Source: CAD feature listing. Evaluate the final solid. Frame: model axes, mm. Face numbers are marked on the shaded views. A direction names the side the tool comes from. Give positions to 0.01 mm unless a question says otherwise; leave off trailing zeros. Order: outer loops, then holes, each group sorted by start corner. A loop starts at its lowest first (then second) coordinate and runs counter-clockwise, first axis right, second up. Notation, with made-up numbers: (-10, 6.25) - (-6, 6.25) arc R3 ccw to (-6, 10.25) - close; hole circle Ø1 at (11, -19). An arc over 180 degrees is marked (long way). Use CSV: the item, a comma, the result in double quotes.
```python
from build123d import *

# Parameters (mm, degrees)
SKETCH_1_W               = 20
SKETCH_1_H               = 10
EXTRUDE_2_DEPTH          = 10
SKETCH_2_W               = 6
SKETCH_2_H               = 2
SKETCH_2_W_2             = 16
SKETCH_2_H_2             = 3
SKETCH_2_W_3             = 1.5
CUT_EXTRUDE_1_DEPTH      = 23.912878475
CUT_EXTRUDE_2_DEPTH      = 20
CUT_EXTRUDE_2_DEPTH_BACK = 20
SKETCH_7_W               = 17
SKETCH_7_H               = 5.873697418


with BuildPart() as part:
    # Эскиз1 → Бобышка-Вытянуть2 (new, symmetric)
    with BuildSketch(Plane.XY):
        Rectangle(SKETCH_1_W, SKETCH_1_H)
    extrude(amount=EXTRUDE_2_DEPTH, both=True)

    # Эскиз2 → Вырез-Вытянуть1 (cut, through all)
    with BuildSketch(Plane.XY.offset(10)):
        with Locations((-7, 4)):
            Rectangle(SKETCH_2_W, SKETCH_2_H)
        Polygon((10, 5), (3, 5), (10, -0.873697418), align=None)
        with Locations((-2, -3.5)):
            Rectangle(SKETCH_2_W_2, SKETCH_2_H_2)
        with Locations((9.25, -4)):
            Rectangle(SKETCH_2_W_3, SKETCH_2_H)
    extrude(amount=-CUT_EXTRUDE_1_DEPTH, mode=Mode.SUBTRACT)

    # Эскиз7 → Вырез-Вытянуть2 (cut, two sides: drawn at the far end of the back side and taken through both)
    with BuildSketch(Plane(origin=(0, 0, 0), x_dir=(0, 0, -1), z_dir=(1, 0, 0)).offset(-CUT_EXTRUDE_2_DEPTH_BACK)):
        with Locations((0, 2.063151291)):
            Rectangle(SKETCH_7_W, SKETCH_7_H)
    extrude(amount=CUT_EXTRUDE_2_DEPTH + CUT_EXTRUDE_2_DEPTH_BACK, mode=Mode.SUBTRACT)


solid = part.part
```
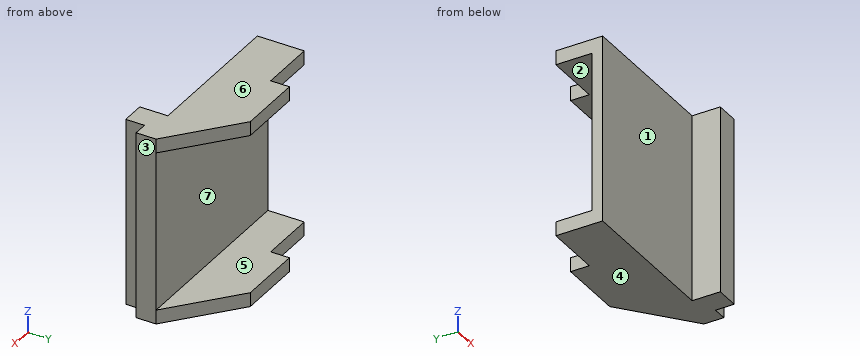
Item 1: Mould query, pull axis Z, two halves, no side actions, for the marked faces 4, 5, 6 and 7. Classes: released by +Z, released by -Z, zero draft, split by the parting line, or undercut.
Filled in:
face 4,"released by -Z"
face 5,"undercut"
face 6,"released by +Z"
face 7,"undercut"
Item 2: First-contact query: pin 1 (5 mm diameter, centred on x = -2.5, z = 3, fed in from +Y); pin 2 (8 mm diameter, centred on x = -1.5, z = 2.5, fed in from -Y); pin 3 (0.8 mm diameter, centred on x = -8, z = 9, fed in from +Y). Flat tips, straight axial feed; report the tip coordinate or a pass-through.
Filled in:
pin 1,"stops at y = -0.87"
pin 2,"stops at y = -2"
pin 3,"stops at y = 3"
Item 3: Section A-A on y = 1.5. Return the cut outline in (x, z).
Filled in:
outline,"(-10, -10) - (7.17, -10) - (7.17, -8.5) - (-10, -8.5) - close; (-10, 8.5) - (7.17, 8.5) - (7.17, 10) - (-10, 10) - close"
Item 4: Section C-C on z = -4.25. Return the cut outline in (x, y), then the cut area to 3 significant figures.
Filled in:
outline,"(-10, -2) - (6, -2) - (6, -5) - (8.5, -5) - (8.5, -3) - (10, -3) - (10, -0.87) - (-10, -0.87) - close"
area,"31.5 mm2"
Item 5: Material intervals for line 1 (Z direction, x = 7, y = -0.25); line 2 (Y direction, x = 7.75, z = -0.25); line 3 (Y direction, x = -8.75, z = 3), sorted ascending. Write a range as from..to.
Filled in:
line 1,"z = -10..-8.5, 8.5..10"
line 2,"y = -5..-0.87"
line 3,"y = -2..-0.87"
Item 6: Section B-B on x = 1. Return the cut outline in (y, z).
Filled in:
outline,"(-2, -10) - (5, -10) - (5, -8.5) - (-0.87, -8.5) - (-0.87, 8.5) - (5, 8.5) - (5, 10) - (-2, 10) - close"
Item 7: Set-up query: the marked faces 1, 2 and 3. Return all of +Z, -Z, +X, -X, +Y, -Y with unobstructed straight access to the full face (end or side cutting, diameter ignored); none if empty.
Filled in:
face 1,"+Z, -Z, -X, -Y"
face 2,"+X, -X, +Y"
face 3,"+Z, -Z, +X, +Y, -Y"
Item 8: Section D-D on y = 0. Return the cut outline in (x, z).
Filled in:
outline,"(-10, -10) - (8.96, -10) - (8.96, -8.5) - (-10, -8.5) - close; (-10, 8.5) - (8.96, 8.5) - (8.96, 10) - (-10, 10) - close"
